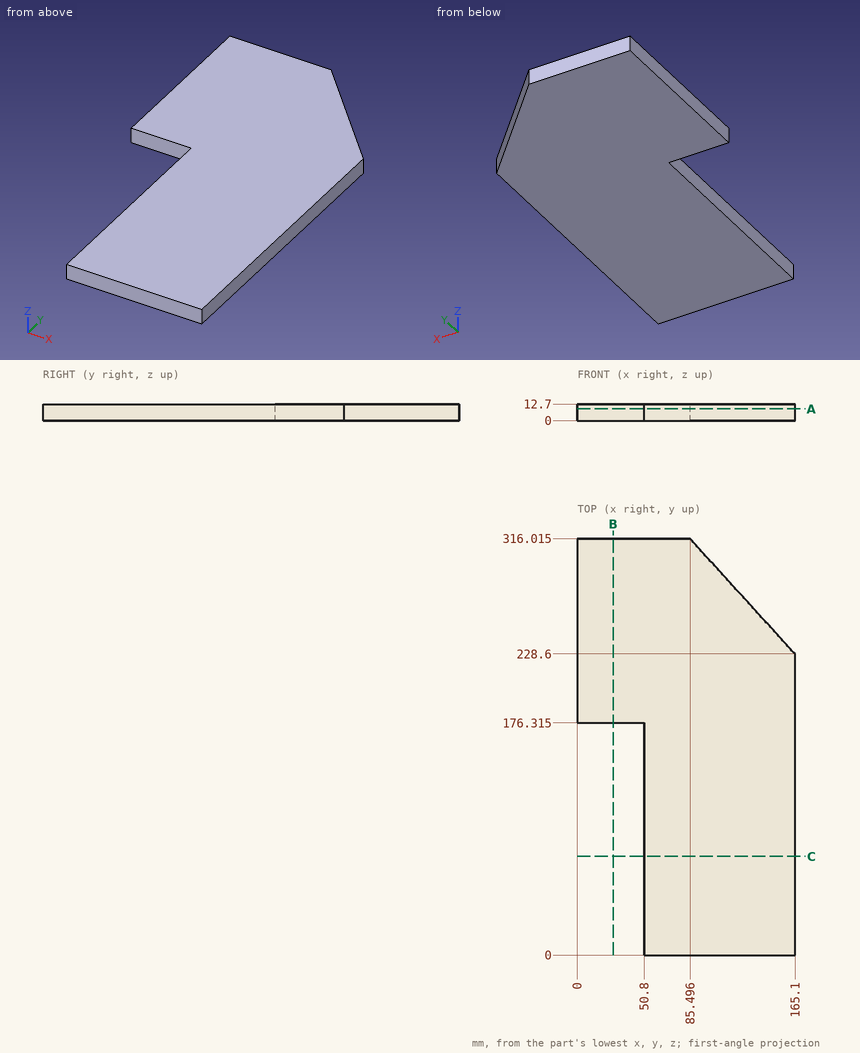
Can you work these out from the drawing? Everything is in mm from the part's minimum corner. Coordinates: 2 decimals unless noted, no trailing zeros. Loops run counter-clockwise (first coordinate to the right, second up) from the corner with the lowest first, then second, coordinate; pieces in that order, holes last.
1. I need wall thicknesses on L1, parallel to Y at x = 23, z = 7.5 (1 decimal); L2, parallel to X at y = 136.5, z = 2.5; L3, parallel to Y at x = 90.5, z = 9. Which ranges of each line are inside material? Lowest first, please.
2. Imagine slicing it at C-C, the plane y = 75. Please give me the cut outline in (x, z).
3. For P1, Ø4, axis at y = 145.5, z = 3, coming from the -X side; P2, Ø4, axis at y = 239, z = 4.5, coming from the +X side, each with a flat end and sliding along its axis, tell me the tip position at first contact or that it passes through.
4. Imagine slicing it at B-B, the plane x = 27. Please give me the cut outline in (y, z) (1 decimal), and give its area (3 significant figures).
5. Imagine slicing it at A-A, the plane z = 9. Please give me the cut outline in (x, y) (1 decimal), and give its area (3 significant figures).
Taken from the geometry:
1. L1: y = 176.3 to 316
1. L2: x = 50.8 to 165.1
1. L3: y = 0 to 310.52
2. outline: (50.8, 0) - (165.1, 0) - (165.1, 12.7) - (50.8, 12.7) - close
3. P1: stops at x = 50.8
3. P2: stops at x = 157.45
4. outline: (176.3, 0) - (316, 0) - (316, 12.7) - (176.3, 12.7) - close
4. area: 1,770 mm2
5. outline: (0, 176.3) - (50.8, 176.3) - (50.8, 0) - (165.1, 0) - (165.1, 228.6) - (85.5, 316) - (0, 316) - close
5. area: 39,700 mm2
